```python
from build123d import *

# Parameters (mm, degrees)
SKETCH_W      = 50
SKETCH_H      = 25
PAD_DEPTH     = 10
SKETCH001_R   = 10
PAD001_DEPTH  = 15
SKETCH002_R   = 2.1
POCKET_DEPTH  = 10
CHAMFER_SIZE2 = 3
CHAMFER_SIZE  = 3


with BuildPart() as part:
    # Sketch → Pad (new body)
    with BuildSketch(Plane.XY):
        with Locations((-25, 12.5)):
            Rectangle(SKETCH_W, SKETCH_H)
    extrude(amount=PAD_DEPTH)

    # Sketch001 → Pad001 (join)
    with BuildSketch(Plane.XY):
        with Locations((-25, 12.5)):
            Circle(SKETCH001_R)
    extrude(amount=PAD001_DEPTH)

    # Sketch002 (on Face9 of Pad001) → Pocket (cut)
    with BuildSketch(Plane.XY.offset(15)):
        with Locations((-25, 12.5)):
            Circle(SKETCH002_R)
    extrude(amount=-POCKET_DEPTH, mode=Mode.SUBTRACT)

    # Chamfer
    chamfer_edges = [part.edges().sort_by_distance(p)[0] for p in [
        (-35, 12.5, 15),
    ]]
    chamfer_side = part.faces().sort_by_distance((-35, 12.5, 12.5))[0]
    chamfer(chamfer_edges, length=CHAMFER_SIZE, length2=CHAMFER_SIZE2, reference=chamfer_side)


solid = part.part
```
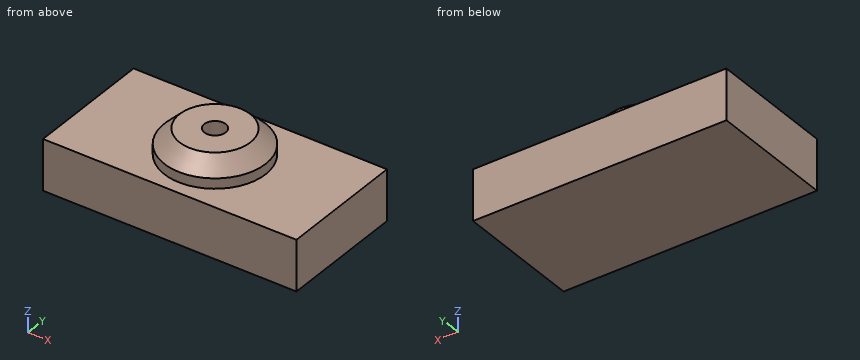
Could you check a few things on this model? Use its own coordinates, in mm. Coordinates: 2 decimals unless noted, no trailing zeros. Order: outer loops, then holes, each group sorted by start corner. A loop starts at its lowest first (then second) coordinate and runs counter-clockwise, first axis right, second up. Notation, with made-up numbers: M 20,-15.75 L 57,-15.75 A11 cw 57,-10.75 Z; hole C 14,25 d11. An arc over 180 degrees is marked long. Use one line per item in the form item = value. Start each with the question number.
1. For pin 1 (2 mm diameter, centred on x = -25, y = 12.5, fed in from +Z), with a flat end and sliding along its axis, tell me the tip position at first contact or that it passes through.
2. Please list where these lines run through material, in increasing order: line 1 (Y direction, x = -25, z = 11.25); line 2 (Y direction, x = -25, z = 7); line 3 (Z direction, x = -40.5, y = 21.5).
3. Suppose I cut it at C-C on z = 12.5. Write out the boundary of the cut face in (x, y), then the cut area to 3 significant figures.
4. Suppose I cut it at A-A on x = -25. Write out the boundary of the cut face in (y, z).
5. Suppose I cut it at B-B on y = 12.5. Write out the boundary of the cut face in (x, z).
Geometry says:
q1.pin_1 = 5
q2.line_1 = 2.5 to 10.4, 14.6 to 22.5
q2.line_2 = 0 to 10.4, 14.6 to 25
q2.line_3 = 0 to 10
q3.outline = C -25,12.5 d19; hole C -25,12.5 d4.2
q3.area = 270 mm^2
q4.outline = M 0,0 L 25,0 L 25,10 L 22.5,10 L 22.5,12 L 19.5,15 L 14.6,15 L 14.6,5 L 10.4,5 L 10.4,15 L 5.5,15 L 2.5,12 L 2.5,10 L 0,10 Z
q5.outline = M -50,0 L 0,0 L 0,10 L -15,10 L -15,12 L -18,15 L -22.9,15 L -22.9,5 L -27.1,5 L -27.1,15 L -32,15 L -35,12 L -35,10 L -50,10 Z
